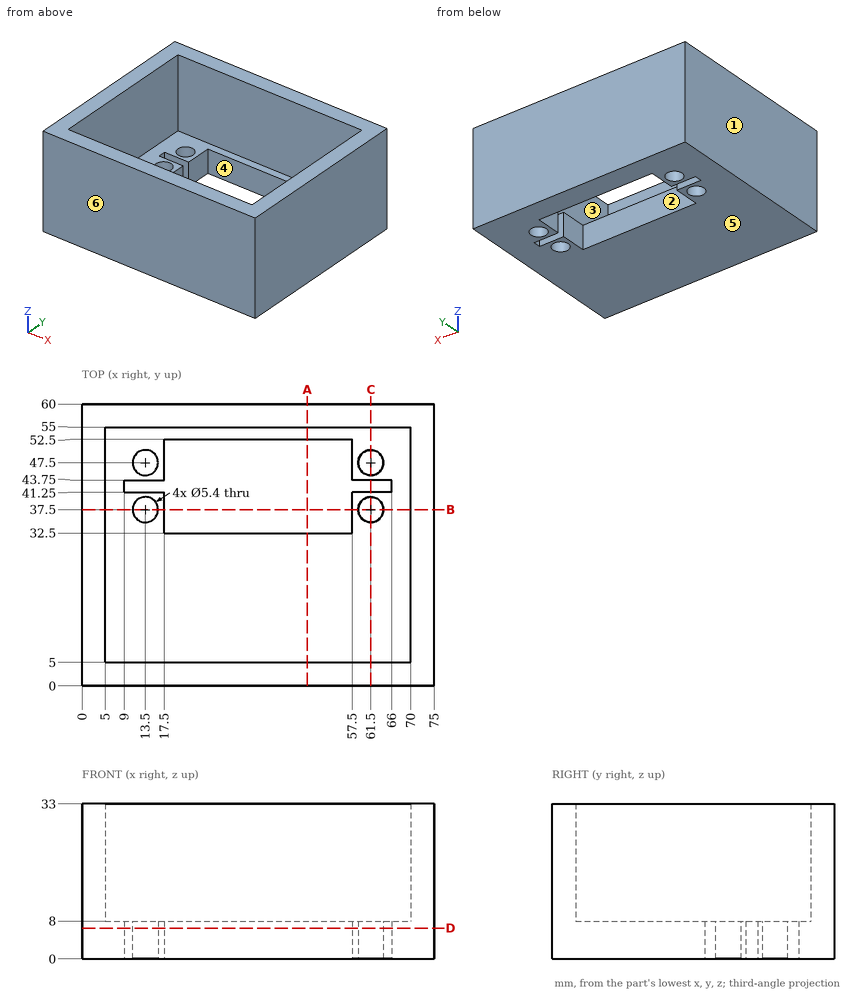
Geometry check sheet. Reference: drawing and pictorial views, mm from the part's lowest x, y, z. A direction names the side the tool comes from. Coordinates: 2 decimals unless noted, no trailing zeros. Order: outer loops, then holes, each group sorted by start corner. A loop starts at its lowest first (then second) coordinate and runs counter-clockwise, first axis right, second up.
Item 1: Section check D-D (z = 6.5). Enter the section's corners in (x, y).
Item 2: Section check C-C (x = 61.5). Enter the section's corners in (y, z).
Item 3: Section check B-B (y = 37.5). Enter the section's corners in (x, z).
Item 4: Section check A-A (x = 48). Enter the section's corners in (y, z), plus the area to 3 significant figures.
Item 5: Depth check by flat-ended pin: pin 1 (3 mm diameter, centred on y = 51, z = 11, fed in from -X); pin 2 (3 mm diameter, centred on x = 13.5, y = 47.5, fed in from +Z). Enter the tip coordinate at first touch or a pass-through.
Item 6: Scan lines: line 1 along Y through (x, z) = (13.5, 1.5); line 2 along X through (y, z) = (26, 17); line 3 along X through (y, z) = (37, 2). Record each from-to range of solid material in increasing order.
Item 7: Mould release check, pull along Y, two halves, no side actions. Record for the marked faces 4, 5 and 6: released by +Y, released by -Y, zero draft, split by the parting line, or undercut.
Item 8: Tool access check on the marked faces 1, 2 and 3. Record the directions out of +Z, -Z, +X, -X, +Y, -Y that give a thin tool (end or side, any length) a straight path to the whole face; none if there is none.
Check sheet entries:
1. outline: (0, 0) - (75, 0) - (75, 60) - (0, 60) - close; hole (9, 41.25) - (17.5, 41.25) - (17.5, 32.5) - (57.5, 32.5) - (57.5, 41.25) - (66, 41.25) - (66, 43.75) - (57.5, 43.75) - (57.5, 52.5) - (17.5, 52.5) - (17.5, 43.75) - (9, 43.75) - close; hole circle Ø5.4 at (13.5, 37.5); hole circle Ø5.4 at (13.5, 47.5); hole circle Ø5.4 at (61.5, 37.5); hole circle Ø5.4 at (61.5, 47.5)
2. outline: (0, 0) - (34.8, 0) - (34.8, 8) - (5, 8) - (5, 33) - (0, 33) - close; (40.2, 0) - (41.25, 0) - (41.25, 8) - (40.2, 8) - close; (43.75, 0) - (44.8, 0) - (44.8, 8) - (43.75, 8) - close; (50.2, 0) - (60, 0) - (60, 33) - (55, 33) - (55, 8) - (50.2, 8) - close
3. outline: (0, 0) - (10.8, 0) - (10.8, 8) - (5, 8) - (5, 33) - (0, 33) - close; (16.2, 0) - (17.5, 0) - (17.5, 8) - (16.2, 8) - close; (57.5, 0) - (58.8, 0) - (58.8, 8) - (57.5, 8) - close; (64.2, 0) - (75, 0) - (75, 33) - (70, 33) - (70, 8) - (64.2, 8) - close
4. outline: (0, 0) - (32.5, 0) - (32.5, 8) - (5, 8) - (5, 33) - (0, 33) - close; (52.5, 0) - (60, 0) - (60, 33) - (55, 33) - (55, 8) - (52.5, 8) - close
4. area: 570 mm2
5. pin 1: stops at x = 0
5. pin 2: passes through
6. line 1: y = 0 to 34.8, 40.2 to 41.25, 43.75 to 44.8, 50.2 to 60
6. line 2: x = 0 to 5, 70 to 75
6. line 3: x = 0 to 10.85, 16.15 to 17.5, 57.5 to 58.85, 64.15 to 75
7. face 4: undercut
7. face 5: zero draft
7. face 6: released by -Y
8. face 1: +Z, -Z, -X, +Y, -Y
8. face 2: +Z, -Z
8. face 3: +Z
